```python
from build123d import *

# Parameters (mm, degrees)
BOSS_EXTRUDE1_DEPTH      = 4.7625
BOSS_EXTRUDE1_DEPTH_BACK = 4.7625
SKETCH2_R                = 1.75
CUT_EXTRUDE1_DEPTH       = 114.796194078
FILLET1_R                = 10
CHAMFER1_SIZE            = 2
CHAMFER2_SIZE            = 1
FILLET2_R                = 3


with BuildPart() as part:
    # Sketch1 → Boss-Extrude1 (new body, two sides)
    with BuildSketch(Plane.XY) as boss_extrude1_sk:
        Polygon((-191.403805922, 11.396194078), (-207.403805922, 27.396194078), (-207.403805922, 57.396194078), (-202.247691321, 62.552308679), (-202.247691321, 125.192388155), (-160.247691321, 125.192388155), (-160.247691321, 119.192388155), (-185.247691321, 119.192388155), (-185.247691321, 14.552308679), (-188.403805922, 11.396194078), align=None)
        with BuildLine():
            Line((-192.497691321, 61.192388155), (-192.497691321, 71.192388155))
            ThreePointArc((-192.497691321, 71.192388155), (-195.247691321, 73.942388155), (-197.997691321, 71.192388155))
            Line((-197.997691321, 71.192388155), (-197.997691321, 61.192388155))
            ThreePointArc((-197.997691321, 61.192388155), (-195.247691321, 58.442388155), (-192.497691321, 61.192388155))
        make_face(mode=Mode.SUBTRACT)
        with BuildLine():
            Line((-192.497691321, 81.192388155), (-192.497691321, 91.192388155))
            ThreePointArc((-192.497691321, 91.192388155), (-195.247691321, 93.942388155), (-197.997691321, 91.192388155))
            Line((-197.997691321, 91.192388155), (-197.997691321, 81.192388155))
            ThreePointArc((-197.997691321, 81.192388155), (-195.247691321, 78.442388155), (-192.497691321, 81.192388155))
        make_face(mode=Mode.SUBTRACT)
        with BuildLine():
            Line((-192.497691321, 101.192388155), (-192.497691321, 111.192388155))
            ThreePointArc((-192.497691321, 111.192388155), (-195.247691321, 113.942388155), (-197.997691321, 111.192388155))
            Line((-197.997691321, 111.192388155), (-197.997691321, 101.192388155))
            ThreePointArc((-197.997691321, 101.192388155), (-195.247691321, 98.442388155), (-192.497691321, 101.192388155))
        make_face(mode=Mode.SUBTRACT)
    extrude(amount=BOSS_EXTRUDE1_DEPTH)
    extrude(boss_extrude1_sk.sketch, amount=-BOSS_EXTRUDE1_DEPTH_BACK)

    # Sketch2 → Cut-Extrude1 (cut, through all)
    with BuildSketch(Plane(origin=(0, 125.192388155, 0), x_dir=(-1, 0, 0), z_dir=(0, 1, 0))):
        with Locations((165.247691321, 0)):
            Circle(SKETCH2_R)
    extrude(amount=-CUT_EXTRUDE1_DEPTH, mode=Mode.SUBTRACT)

    # Fillet1
    fillet1_edges = [part.edges().sort_by_distance(p)[0] for p in [
        (-202.247691321, 62.552308679, 0),
    ]]
    fillet(fillet1_edges, radius=FILLET1_R)

    # Chamfer1
    chamfer1_edges = [part.edges().sort_by_distance(p)[0] for p in [
        (-202.247691321, 125.192388155, 0),
    ]]
    chamfer(chamfer1_edges, length=CHAMFER1_SIZE)

    # Chamfer2
    chamfer2_edges = [part.edges().sort_by_distance(p)[0] for p in [
        (-160.247691321, 125.192388155, 0),
        (-160.247691321, 119.192388155, 0),
    ]]
    chamfer(chamfer2_edges, length=CHAMFER2_SIZE)

    # Fillet2
    fillet2_edges = [part.edges().sort_by_distance(p)[0] for p in [
        (-185.247691321, 119.192388155, 0),
    ]]
    fillet(fillet2_edges, radius=FILLET2_R)


solid = part.part
```
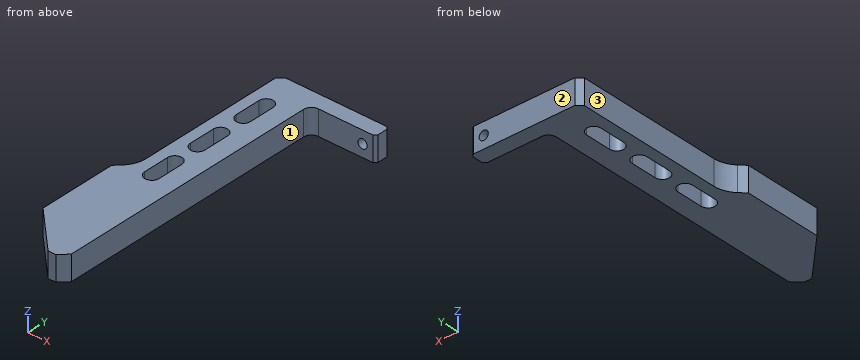
Design review of the part built by this model. Coordinates are the model's own, in mm. Face numbers are marked on the shaded views. A direction names the side the tool comes from. Give positions to 0.01 mm unless a question says otherwise; leave off trailing zeros. Order: outer loops, then holes, each group sorted by start corner. A loop starts at its lowest first (then second) coordinate and runs counter-clockwise, first axis right, second up. Notation, with made-up numbers: (21, 78) -> (40, 78) arc R11 ccw to (40, 95) -> close; hole circle Ø3 at (83, -32). An arc over 180 degrees is marked (long way). Write item = value, one per line. Start each with the question number.
(1) For pin 1 (3 mm diameter, centred on y = 67.5, z = -0.5, fed in from +X); pin 2 (5 mm diameter, centred on y = 105, z = 1, fed in from -X); pin 3 (3 mm diameter, centred on x = -171.5, z = -1, fed in from -Y), all flat-tipped, find the tip position at first contact; note any pin that passes through.
(2) We need section C-C on y = 43. Write out the cut boundary in (x, z), plus the area to 3 significant figures.
(3) We need section B-B on x = -195. Write out the cut boundary in (y, z).
(4) We need section A-A on z = 0. State how many separate pieces and enclosed holes the cut face has, plus the area to 3 significant figures.
(5) To check wall thickness, follow line 1 along Y through (x, z) = (-197, 1.75); line 2 along X through (y, z) = (104, 3.5); line 3 along X through (y, z) = (112, -3.75). State the ranges of each line that lie inside material, in increasing order.
(6) We need section D-D on x = -181. Write out the cut boundary in (y, z).
(7) For the marked faces 1, 2 and 3, list the 3-axis set-ups (+Z, -Z, +X, -X, +Y, -Y) from which the entire face can be reached by the end or side of a thin tool; tool diameter is ignored.
Numbers:
q1.pin_1 = -185.25
q1.pin_2 = -202.25
q1.pin_3 = 119.19
q2.outline = (-207.4, -4.76) -> (-185.25, -4.76) -> (-185.25, 4.76) -> (-207.4, 4.76) -> close
q2.area = 211 mm^2
q3.outline = (14.99, -4.76) -> (58.45, -4.76) -> (58.45, 4.76) -> (14.99, 4.76) -> close; (73.93, -4.76) -> (78.45, -4.76) -> (78.45, 4.76) -> (73.93, 4.76) -> close; (93.93, -4.76) -> (98.45, -4.76) -> (98.45, 4.76) -> (93.93, 4.76) -> close; (113.93, -4.76) -> (125.19, -4.76) -> (125.19, 4.76) -> (113.93, 4.76) -> close
q4.separate_pieces = 2
q4.enclosed_holes = 3
q4.area = 1,950 mm^2
q5.line_1 = 16.99 to 59.07, 73.31 to 79.07, 93.31 to 99.07, 113.31 to 125.19
q5.line_2 = -202.25 to -198, -192.5 to -185.25
q5.line_3 = -202.25 to -197.88, -192.62 to -185.25
q6.outline = (119.19, -4.76) -> (125.19, -4.76) -> (125.19, 4.76) -> (119.19, 4.76) -> close
q7.face_1 = +Z, -Z, +X, -Y
q7.face_2 = +Z, -Z, +X, -X, +Y
q7.face_3 = +Z, -Z, -X, +Y
